from build123d import *

# Parameters (mm, degrees)
F1_DEPTH = 19.05
F2_W     = 46.99
F2_H     = 15.24
F3_DEPTH = 50.801
F4_R     = 2.15265
F5_DEPTH = 3.811
F6_R     = 2.54
F7_R     = 6.132068


with BuildPart() as f1:
    # F0 (on Top) → F1 (new body)
    with BuildSketch(Plane.XY):
        Polygon((38.1, 15.24), (38.1, 35.56), (50.8, 35.56), (50.8, 50.8), (0, 50.8), (0, 0), (50.8, 0), (50.8, 15.24), align=None)
    extrude(amount=F1_DEPTH)

    # F2 (on face) → F3 (cut, through all)
    with BuildSketch(Plane(origin=(0, 50.8, 0), x_dir=(-1, 0, 0), z_dir=(0, 1, 0))):
        with Locations((-27.305, 11.43)):
            Rectangle(F2_W, F2_H)
    extrude(amount=-F3_DEPTH, mode=Mode.SUBTRACT)

    # F4 (on face) → F5 (cut, through all)
    with BuildSketch(Plane.YZ.offset(3.81)):
        with Locations((38.1, 11.43)):
            Circle(F4_R)
        with Locations((12.7, 11.43)):
            Circle(F4_R)
    extrude(amount=-F5_DEPTH, mode=Mode.SUBTRACT)

    # F6
    f6_edges = [f1.edges().sort_by_distance(p)[0] for p in [
        (3.81, 25.4, 3.81),
    ]]
    fillet(f6_edges, radius=F6_R)

    # F7
    f7_edges = [f1.edges().sort_by_distance(p)[0] for p in [
        (0, 25.4, 0),
    ]]
    fillet(f7_edges, radius=F7_R)


solid = f1.part
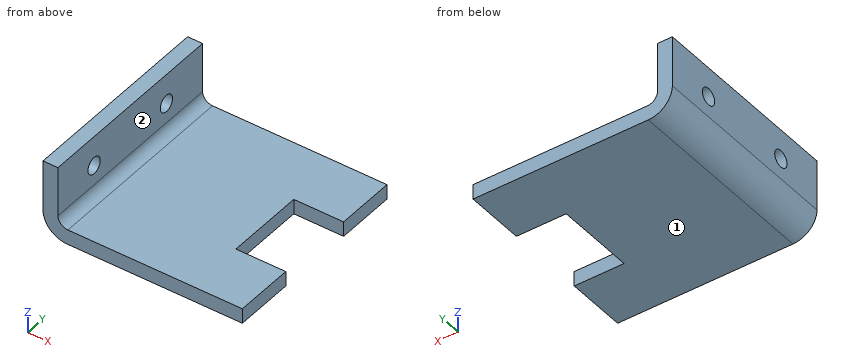
Work out the finished part from the listing and answer in its coordinate system (mm). Face numbers are marked on the shaded views. A direction names the side the tool comes from. Give positions to 0.01 mm unless a question says otherwise; leave off trailing zeros. Order: outer loops, then holes, each group sorted by start corner. A loop starts at its lowest first (then second) coordinate and runs counter-clockwise, first axis right, second up. Notation, with made-up numbers: (58.25, -12.75) -> (108.25, -12.75) arc R28 ccw to (108.25, 7.25) -> close; hole circle Ø8 at (81, -24). An arc over 180 degrees is marked (long way). Answer as a JSON object with one key per item and string values. Group by question number.
1. Section B-B on z = 11.43 is taken. Determine the outline of the cut face in (x, y), plus the area to 3 significant figures.
2. Section C-C on y = 8 is taken. Determine the outline of the cut face in (x, z).
3. Flat-ended cylindrical pins translate along their axes: pin 1 Ø10 at (x, z) = (16, 4) entering from -Y; pin 2 Ø3 at (y, z) = (13.5, 8.5) entering from +X; pin 3 Ø1.1 at (y, z) = (29, 2) entering from +X; pin 4 Ø8 at (x, y) = (43, 16) entering from +Z. Find the tip coordinate at first contact, or state that the pin passes through.
4. Section A-A on y = 38.1 is taken. Determine the outline of the cut face in (x, z).
5. Consider line 1 along Z through (x, y) = (23, 5); line 2 along Z through (x, y) = (1, 38). Determine where each line is inside the solid, lowest interval first. Write a range as [from, to].
6. Section D-D on z = 1.5 is taken. Determine the outline of the cut face in (x, y), plus the area to 3 significant figures.
7. A tool of negligible diameter and unlimited length cuts with its end or side. For the marked faces 1 and 2, from which of +Z, -Z, +X, -X, +Y, -Y can it reach the whole face along a straight path? Write none if from no direction.
Result sheet:
{
 "1": {"outline": "(0, 0) -> (3.81, 0) -> (3.81, 10.55) -> (0, 10.55) -> close; (0, 14.85) -> (3.81, 14.85) -> (3.81, 35.95) -> (0, 35.95) -> close; (0, 40.25) -> (3.81, 40.25) -> (3.81, 50.8) -> (0, 50.8) -> close", "area": "161 mm^2"},
 "2": {"outline": "(0, 6.13) arc R6.13 ccw to (6.13, 0) -> (50.8, 0) -> (50.8, 3.81) -> (6.35, 3.81) arc R2.54 cw to (3.81, 6.35) -> (3.81, 19.05) -> (0, 19.05) -> close"},
 "3": {"pin 1": "stops at y = 0", "pin 2": "stops at x = 3.81", "pin 3": "stops at x = 38.1", "pin 4": "stops at z = 3.81"},
 "4": {"outline": "(0, 6.13) arc R6.13 ccw to (6.13, 0) -> (50.8, 0) -> (50.8, 3.81) -> (6.35, 3.81) arc R2.54 cw to (3.81, 6.35) -> (3.81, 9.28) -> (0, 9.28) -> close; (0, 13.58) -> (3.81, 13.58) -> (3.81, 19.05) -> (0, 19.05) -> close"},
 "5": {"line 1": "z = [0, 3.81]", "line 2": "z = [2.78, 9.28], [13.58, 19.05]"},
 "6": {"outline": "(2.11, 0) -> (50.8, 0) -> (50.8, 15.24) -> (38.1, 15.24) -> (38.1, 35.56) -> (50.8, 35.56) -> (50.8, 50.8) -> (2.11, 50.8) -> close", "area": "2,220 mm^2"},
 "7": {"face 1": "-Z, +X, -X, +Y, -Y", "face 2": "+Z, +X, +Y, -Y"}
}
